```python
from build123d import *

# Parameters (mm, degrees)
SKETCH2_R                  = 25.7
BOSS_EXTRUDE1_DEPTH        = 2
SKETCH3_W                  = 14.6
SKETCH3_H                  = 5.6
CUT_EXTRUDE1_DEPTH         = 37.400274724
F_1_6_1_6_DIAMETER_HOLE1_D = 1.6


with BuildPart() as part:
    # Sketch2 → Boss-Extrude1 (new body)
    with BuildSketch(Plane(origin=(0, 0, 0), x_dir=(1, 0, 0), z_dir=(0, 1, 0))):
        with Locations(Location((0, 0, 0), (0, 0, 270))):
            Circle(SKETCH2_R)
    extrude(amount=BOSS_EXTRUDE1_DEPTH)

    # Sketch3 → Cut-Extrude1 (cut, through all)
    with BuildSketch(Plane(origin=(0, 2, 0), x_dir=(1, 0, 0), z_dir=(0, 1, 0))):
        Rectangle(SKETCH3_W, SKETCH3_H)
    extrude(amount=-CUT_EXTRUDE1_DEPTH, mode=Mode.SUBTRACT)

    # Ø1.6 (1.6) Diameter Hole1 (through all)
    with Locations(Plane(origin=(-10.1, 2, -1), x_dir=(0, 0, 1), z_dir=(0, 1, 0))):
        with Locations((0, 0), (2, 26.6)):
            Hole(F_1_6_1_6_DIAMETER_HOLE1_D / 2)


solid = part.part
```
Model file for the job. Use its own axes, mm. A direction names the side the tool comes from. Coordinates: 2 decimals unless noted, no trailing zeros. Loops run counter-clockwise (first coordinate to the right, second up) from the corner with the lowest first, then second, coordinate; pieces in that order, holes last. Notation, with made-up numbers: (-31.5, 6) - (-12.5, 6) arc R35 ccw to (-12.5, 39) - close; hole circle Ø10 at (80, -11). An arc over 180 degrees is marked (long way). Write item = value, one per line. Start each with the question number.
Item 1: Pull direction Z, two halves, no side cores. Call faces 1 (the face through (-25.09, 0.99, -5.57)), 2 (the face through (0, 1, 2.8)), 3 (the face through (0, 0, 5)): +Z half, -Z half, draft (parallel to the pull), parting line (faces both ways), or undercut.
Item 2: Drop flat-ended pins along their axis: pin 1 Ø0.6 at (x, y) = (3.5, 1) entering from +Z; pin 2 Ø8 at (x, z) = (13.5, 1.5) entering from -Y; pin 3 Ø1 at (x, y) = (15.5, 1) entering from +Z; pin 4 Ø1 at (x, z) = (16.5, 1) entering from -Y. Give the stop position or say it passes through.
Item 3: Saw through at B-B, the plane y = 1.15. List the corners of the cut face in (x, z).
Item 4: Saw through at C-C, the plane z = -1. List the corners of the cut face in (x, y).
Item 5: Saw through at A-A, the plane x = 0. List the corners of the cut face in (y, z).
Item 6: Wall check: probe 1 along X at (y, z) = (1.95, 0); probe 2 along X at (y, z) = (0.4, 1); probe 3 along Z at (x, y) = (-6, 0.7). Give the ranges that are in metal, low to high. Write a range as [from, to].
Item 7: 3-axis set-ups, long thin cutter, end or side, ignore diameter. For faces 4 (the face through (-7.3, 1, 0)), 5 (the face through (0, 2, 5)): which of +Z, -Z, +X, -X, +Y, -Y reach the whole face in a straight line?
Item 8: Saw through at D-D, the plane x = -10.1. List the corners of the cut face in (y, z).
Answers:
q1.face_1 = parting line
q1.face_2 = undercut
q1.face_3 = draft
q2.pin_1 = 25.5
q2.pin_2 = 0
q2.pin_3 = 20.87
q2.pin_4 = through
q3.outline = circle Ø51.4 at (0, 0); hole circle Ø1.6 at (-10.1, -1); hole (-7.3, -2.8) - (7.3, -2.8) - (7.3, 2.8) - (-7.3, 2.8) - close; hole circle Ø1.6 at (16.5, 1)
q4.outline = (-25.68, 0) - (-10.9, 0) - (-10.9, 2) - (-25.68, 2) - close; (-9.3, 0) - (-7.3, 0) - (-7.3, 2) - (-9.3, 2) - close; (7.3, 0) - (25.68, 0) - (25.68, 2) - (7.3, 2) - close
q5.outline = (0, -25.7) - (2, -25.7) - (2, -2.8) - (0, -2.8) - close; (0, 2.8) - (2, 2.8) - (2, 25.7) - (0, 25.7) - close
q6.probe_1 = [-25.7, -7.3], [7.3, 25.7]
q6.probe_2 = [-25.68, -7.3], [7.3, 15.7], [17.3, 25.68]
q6.probe_3 = [-24.99, -2.8], [2.8, 24.99]
q7.face_4 = +Y, -Y
q7.face_5 = +Z, -Z, +X, -X, +Y
q8.outline = (0, -23.63) - (2, -23.63) - (2, -1.8) - (0, -1.8) - close; (0, -0.2) - (2, -0.2) - (2, 23.63) - (0, 23.63) - close
